Source: three-view drawing plus pictorial views. Frame: mm from the lowest corner of the part. A direction names the side the tool comes from. Round coordinates to 2 decimals unless told otherwise and drop trailing zeros. Loops run counter-clockwise (first coordinate to the right, second up) from the corner with the lowest first, then second, coordinate; pieces in that order, holes last. Notation, with made-up numbers: (-16, -11) -> (18, -11) arc R11 ccw to (18, 6) -> close; hole circle Ø7 at (35.25, 66.5). An arc over 180 degrees is marked (long way). Answer in a Markdown table with one row per item.
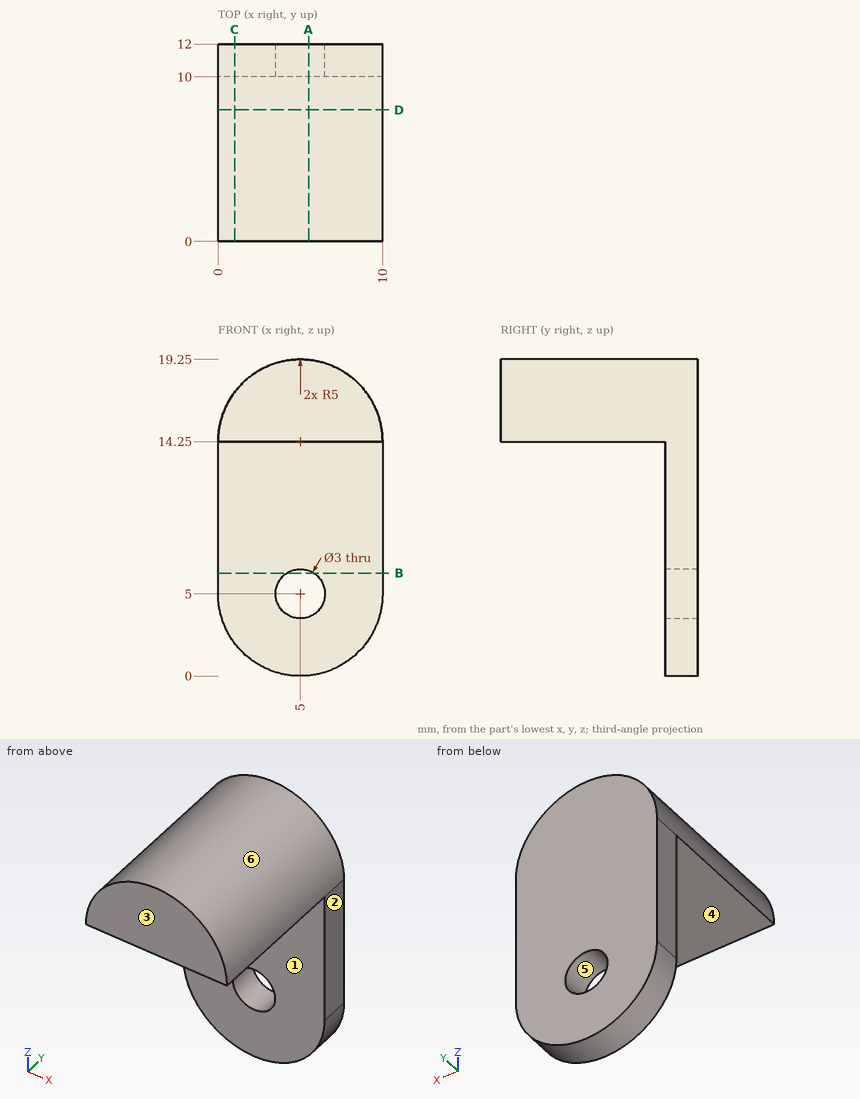
Item 1: Reachability of the marked faces 1 and 2 from +Z, -Z, +X, -X, +Y, -Y: full face, straight path, thin tool, end or side. Return the list, or none.
Answer:
| item | result |
|---|---|
| face 1 | -Z, +X, -X, -Y |
| face 2 | +Z, -Z, +X, +Y, -Y |
Item 2: Cut plane D-D (y = 8). Output: boundary loops of the cut face in (x, z).
Answer:
| item | result |
|---|---|
| outline | (0, 14.25) -> (10, 14.25) arc R5 ccw to start |
Item 3: Cut plane A-A (x = 5.5). Output: boundary loops of the cut face in (y, z), then the cut area to 3 significant figures.
Answer:
| item | result |
|---|---|
| outline | (0, 14.25) -> (10, 14.25) -> (10, 6.41) -> (12, 6.41) -> (12, 19.22) -> (0, 19.22) -> close; (10, 0.03) -> (12, 0.03) -> (12, 3.59) -> (10, 3.59) -> close |
| area | 82.5 mm² |
Item 4: Draft query along Z for the marked faces 3, 4, 5 and 6. Return one class per face: pulls with the +Z half, pulls with the -Z half, needs draft (parallel to the pull), parting line crosses it, or undercut.
Answer:
| item | result |
|---|---|
| face 3 | needs draft |
| face 4 | pulls with the -Z half |
| face 5 | undercut |
| face 6 | pulls with the +Z half |
Item 5: Cut plane B-B (z = 6.25). Output: boundary loops of the cut face in (x, y).
Answer:
| item | result |
|---|---|
| outline | (0, 10) -> (4.17, 10) -> (4.17, 12) -> (0, 12) -> close; (5.83, 10) -> (10, 10) -> (10, 12) -> (5.83, 12) -> close |
Item 6: Cut plane C-C (x = 1). Output: boundary loops of the cut face in (y, z), then the cut area to 3 significant figures.
Answer:
| item | result |
|---|---|
| outline | (0, 14.25) -> (10, 14.25) -> (10, 2) -> (12, 2) -> (12, 17.25) -> (0, 17.25) -> close |
| area | 60.5 mm² |
Item 7: Line query: probe 1 along X at (y, z) = (11.05, 5); probe 2 along Y at (x, z) = (7.75, 7); probe 3 along Z at (x, y) = (8, 8.5). Output: solid intervals per line, ascending. Write a range as [from, to].
Answer:
| item | result |
|---|---|
| probe 1 | x = [0, 3.5], [6.5, 10] |
| probe 2 | y = [10, 12] |
| probe 3 | z = [14.25, 18.25] |
Item 8: Pin query (flat end, axial travel): pin 1 Ø1 at (y, z) = (9, 16) entering from +X; pin 2 Ø2 at (x, z) = (1.5, 2.5) entering from -Y; pin 3 Ø3 at (x, y) = (2.5, 3.5) entering from +Z. Return the tip coordinate at first contact, or that it passes through.
Answer:
| item | result |
|---|---|
| pin 1 | stops at x = 9.84 |
| pin 2 | stops at y = 10 |
| pin 3 | stops at z = 19.15 |
